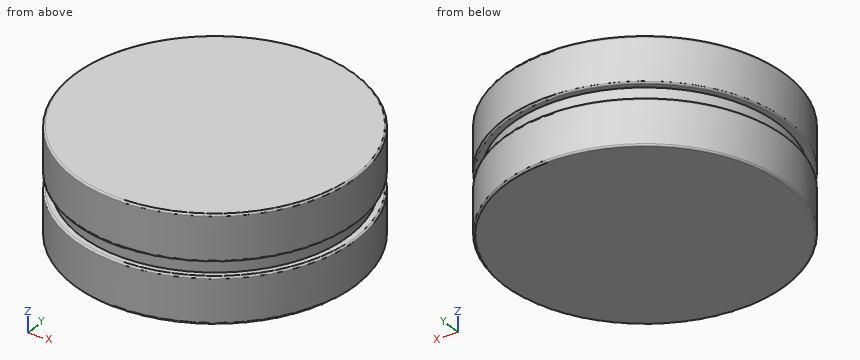
Autodesk Inventor part; units mm, degrees
ref_plane "Work Plane1" through (0, 0, 6.5) normal (0, 0, 1) x (1, 0, 0)
ref_plane "YZ Plane" through (0, 0, 0) normal (1, 0, 0) x (0, 1, 0)
ref_plane "XZ Plane" through (0, 0, 0) normal (0, 1, 0) x (-1, 0, 0)
sketch "Sketch1" plane through (0, 0, 0) normal (0, 0, 1) x (1, 0, 0)
  circle A0 centre (0, 0) radius 20
  dimension "d0" = 40
extrude "Extrusion1" add sketch "Sketch1" along normal blind 15
ref_plane "Work Plane1" through (0, 0, 6.5) normal (0, 0, 1) x (1, 0, 0)
sketch "Sketch2" plane through (0, 0, 6.5) normal (0, 0, 1) x (1, 0, 0)
  circle A0 centre (0, 0) radius 20
  circle A1 centre (0, 0) radius 20
  circle A2 centre (0, 0) radius 19
  dimension "d4" = 38
extrude "Extrusion2" cut sketch "Sketch2" along normal blind 2
fillet "Fillet1" radius 0.25 4 edges at (-20, 0, 6.5) (-20, 0, 8.5) (-20, 0, 0) (-20, 0, 15)
properties part number "Encoder Mount Hole Plug"
Check sheet for the modelled part. Datum: model origin and axes. Units: mm. Round coordinates to 2 decimals unless told otherwise and drop trailing zeros. Loops run counter-clockwise (first coordinate to the right, second up) from the corner with the lowest first, then second, coordinate; pieces in that order, holes last. Notation, with made-up numbers: M -31.5,-33 L -15.5,-33 A21 cw -15.5,-3 Z; hole C 69,26 d1. An arc over 180 degrees is marked long. Answer as a JSON object with one key per item and string values.
1. Scan lines: line 1 (Z direction, x = -10, y = 17); line 2 (X direction, y = 11, z = 3.75); line 3 (X direction, y = 8, z = 5.5). Record each from-to range of solid material in increasing order.
Reply:
{"line 1": "z = 0 to 6.5, 8.5 to 15", "line 2": "x = -16.7 to 16.7", "line 3": "x = -18.33 to 18.33"}
2. Gauge pin test, flat ends, axial feed: P1, Ø1.5, axis at y = 3.5, z = 7, coming from the +X side; P2, Ø4, axis at y = 11.5, z = 4, coming from the +X side; P3, Ø8, axis at x = -1, z = 10, coming from the +Y side. Record the tip position at first contact, or that the pin passes through.
Reply:
{"P1": "stops at x = 19.74", "P2": "stops at x = 17.6", "P3": "stops at y = 20"}
3. Section check A-A (z = 3.25). Record the boundary of the cut face in (x, y).
Reply:
{"outline": "C 0,0 d40"}
4. Section check B-B (z = 7). Record the boundary of the cut face in (x, y).
Reply:
{"outline": "C 0,0 d38"}
